from build123d import *

# Parameters (mm, degrees)
FILLET1_R          = 0.254
CUT_EXTRUDE1_DEPTH = 3.81


with BuildPart() as part:
    # Sketch1 → Revolve1 (revolve)
    with BuildSketch(Plane.XY, mode=Mode.PRIVATE) as revolve1_sk:
        Polygon((2.159, 0), (2.159, 4.826), (3.4925, 4.826), (3.4925, 8.636), (0, 8.636), (0, 0), align=None)
    revolve(revolve1_sk.sketch.rotate(Axis((0, 0, 0), (0, -1, 0)), 90), axis=Axis((0, 0, 0), (0, -1, 0)))

    # Fillet1
    fillet1_edges = [part.edges().sort_by_distance(p)[0] for p in [
        (0, 8.636, -3.4925),
        (0, 4.826, -3.4925),
    ]]
    fillet(fillet1_edges, radius=FILLET1_R)

    # Sketch2 → Cut-Extrude1 (cut)
    with BuildSketch(Plane(origin=(0, 8.636, 0), x_dir=(1, 0, 0), z_dir=(0, 1, 0))):
        Polygon((1.099852263, 1.905), (-1.099852263, 1.905), (-2.199704526, 0), (-1.099852263, -1.905), (1.099852263, -1.905), (2.199704526, 0), align=None)
    extrude(amount=-CUT_EXTRUDE1_DEPTH, mode=Mode.SUBTRACT)


solid = part.part
The listing builds one solid part. Answer for the finished solid, in the listing's coordinates (mm). A direction names the side the tool comes from. Give positions to 0.01 mm unless a question says otherwise; leave off trailing zeros. Write each loop counter-clockwise with the first axis right and the second up, starting at its lowest first coordinate (ties: lowest second). Pieces come first, ordered by that corner, then holes.
Item 1: Section A-A, the plane y = 5.5 is taken. Write down the section's boundary in (x, z) (1 decimal), plus the area to 3 significant figures.
Item 2: Determine the mould class of faces 1 (the flat face through (0, 8.636, 2.1)), 2 (the flat face through (0, 4.826, 0)), 3 (the cylindrical face through (-2.14, 2.45, -0.28)) for opening direction Z: released by +Z, released by -Z, zero draft, split by the parting line, or undercut.
Item 3: Flat-ended cylindrical pins translate along their axes: P1, Ø2, axis at x = 2.5, y = 5.5, coming from the -Z side; P2, Ø4, axis at y = 2.5, z = 2, coming from the -X side; P3, Ø2, axis at x = -0.5, y = 1.5, coming from the +Z side; P4, Ø4, axis at x = -0.5, z = 0.5, coming from the +Y side. Find the tip coordinate at first contact, or state that the pin passes through.
Item 4: Find the intervals of material crossed by line 1 along Y through (x, z) = (-1.75, -0.5); line 2 along Z through (x, y) = (-0.25, 7.5) (3 decimals); line 3 along X through (y, z) = (5.75, -0.25), in increasing order.
Item 5: Section C-C, the plane y = 0.5 is taken. Write down the section's boundary in (x, z).
Item 6: Which of the six approach directions +Z, -Z, +X, -X, +Y, -Y give full straight-line access (tool end or side, diameter ignored) to faces 4 (the flat face through (0, 0, 0)), 5 (the flat face through (-1.64, 6.76, -0.97))?
Completed:
1. outline: circle Ø7 at (0, 0); hole (-2.2, 0) - (-1.1, -1.9) - (1.1, -1.9) - (2.2, 0) - (1.1, 1.9) - (-1.1, 1.9) - close
1. area: 25.7 mm2
2. face 1: zero draft
2. face 2: undercut
2. face 3: split by the parting line
3. P1: stops at z = -3.15
3. P2: stops at x = -2.16
3. P3: stops at z = 2.16
3. P4: stops at y = 8.64
4. line 1: y = 0 to 4.83
4. line 2: z = -3.484 to -1.905, 1.905 to 3.484
4. line 3: x = -3.48 to -2.06, 2.06 to 3.48
5. outline: circle Ø4.32 at (0, 0)
6. face 4: +Z, -Z, +X, -X, -Y
6. face 5: +Y
